Work out the finished part from the listing and answer in its coordinate system (mm). Face numbers are marked on the shaded views. A direction names the side the tool comes from. Give positions to 0.01 mm unless a question says otherwise; leave off trailing zeros. Order: outer loops, then holes, each group sorted by start corner. A loop starts at its lowest first (then second) coordinate and runs counter-clockwise, first axis right, second up.
```python
from build123d import *

# Parameters (mm, degrees)
EXTRUDE_1_DEPTH     = 5.5
SKETCH_2_R          = 1.7
EXTRUDE_2_DEPTH     = 2
SKETCH_3_R          = 2
EXTRUDE_3_DEPTH     = 9
SKETCH_4_R          = 2.5
EXTRUDE_4_DEPTH     = 2
SKETCH_5_R          = 2
EXTRUDE_5_DEPTH     = 16
SKETCH_6_R          = 2.1
EXTRUDE_6_DEPTH     = 1
CHAMFER_1_SIZE      = 0.5
SKETCH_7_W          = 5
SKETCH_7_H          = 0.8
CUT_EXTRUDE_1_DEPTH = 6


with BuildPart() as part:
    # 草图1 → 凸台-拉伸1 (new body)
    with BuildSketch(Plane(origin=(0, 0, 0), x_dir=(0, 0, -1), z_dir=(1, 0, 0))):
        Polygon((-2, 0), (-1, -1.732050808), (1, -1.732050808), (2, 0), (1, 1.732050808), (-1, 1.732050808), align=None)
    extrude(amount=EXTRUDE_1_DEPTH)

    # 草图2 → 凸台-拉伸2 (add)
    with BuildSketch(Plane(origin=(5.5, 0, 0), x_dir=(0, 0, -1), z_dir=(1, 0, 0))):
        Circle(SKETCH_2_R)
    extrude(amount=EXTRUDE_2_DEPTH)

    # 草图3 → 凸台-拉伸3 (add)
    with BuildSketch(Plane(origin=(7.5, 0, 0), x_dir=(0, 0, -1), z_dir=(1, 0, 0))):
        Circle(SKETCH_3_R)
    extrude(amount=EXTRUDE_3_DEPTH)

    # 草图4 → 凸台-拉伸4 (add)
    with BuildSketch(Plane(origin=(16.5, 0, 0), x_dir=(0, 0, -1), z_dir=(1, 0, 0))):
        Circle(SKETCH_4_R)
    extrude(amount=EXTRUDE_4_DEPTH)

    # 草图5 → 凸台-拉伸5 (add)
    with BuildSketch(Plane(origin=(18.5, 0, 0), x_dir=(0, 0, -1), z_dir=(1, 0, 0))):
        Circle(SKETCH_5_R)
    extrude(amount=EXTRUDE_5_DEPTH)

    # 草图6 → 凸台-拉伸6 (add)
    with BuildSketch(Plane(origin=(34.5, 0, 0), x_dir=(0, 0, -1), z_dir=(1, 0, 0))):
        Circle(SKETCH_6_R)
    extrude(amount=-EXTRUDE_6_DEPTH)

    # 倒角1
    chamfer_1_edges = [part.edges().sort_by_distance(p)[0] for p in [
        (34.5, 0, 2.1),
    ]]
    chamfer(chamfer_1_edges, length=CHAMFER_1_SIZE)

    # 草图7 → 切除-拉伸1 (cut)
    with BuildSketch(Plane(origin=(34.5, 0, 0), x_dir=(0, 0, -1), z_dir=(1, 0, 0))):
        Rectangle(SKETCH_7_W, SKETCH_7_H)
    extrude(amount=-CUT_EXTRUDE_1_DEPTH, mode=Mode.SUBTRACT)


solid = part.part
```
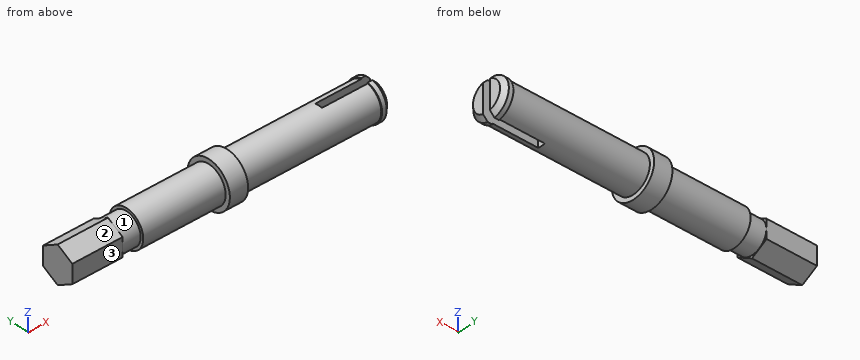
1. Straight lines are drawn through the part: probe 1 along Z at (x, y) = (9, 0.05); probe 2 along X at (y, z) = (1.45, -1.1); probe 3 along Y at (x, z) = (2.5, 0.35). For each, find the intervals that lie inside material, in ascending order.
Findings below:
probe 1: z = -2 to 2
probe 2: x = 0 to 5.5, 7.5 to 34.28
probe 3: y = -1.73 to 1.73
2. The part is cut by section C-C (x = 17.5). Write down the section's boundary in (y, z).
Findings below:
outline: circle Ø5 at (0, 0)
3. The part is cut by section A-A (x = 4.5). Write down the section's boundary in (y, z).
Findings below:
outline: (-1.73, -1) - (0, -2) - (1.73, -1) - (1.73, 1) - (0, 2) - (-1.73, 1) - close
4. Which of the six approach directions +Z, -Z, +X, -X, +Y, -Y give full straight-line access (tool end or side, diameter ignored) to the marked faces 1, 2 and 3?
Findings below:
face 1: none
face 2: +Z, -X, -Y
face 3: +Z, -Z, -X, -Y
5. Given P1, Ø2, axis at x = 3.5, z = 0.5, coming from the -Y side; P2, Ø2, axis at x = 4, z = 0, coming from the +Y side; P3, Ø2, axis at x = 17, y = 1.5, coming from the +Z side, each flat-ended and moving along its own axis, determine where each tip first touches the part or whether it passes through.
Findings below:
P1: stops at y = -1.73
P2: stops at y = 1.73
P3: stops at z = 2.45
6. The part is cut by section D-D (x = 21.5). Write down the section's boundary in (y, z).
Findings below:
outline: circle Ø4 at (0, 0)
